from build123d import *

# Parameters (mm, degrees)
F0_W     = 105
F0_H     = 50
F0_R     = 6
F1_DEPTH = 15
F2_R     = 3
F3_DEPTH = 15
F4_R     = 2.6
F5_DEPTH = 15


with BuildPart() as f1:
    # F0 (on Front) → F1 (new body)
    with BuildSketch(Plane.XZ):
        with Locations((52.5, 25)):
            Rectangle(F0_W, F0_H)
        with Locations((14, 12.5)):
            Circle(F0_R, mode=Mode.SUBTRACT)
        with Locations((91, 12.5)):
            Circle(F0_R, mode=Mode.SUBTRACT)
        with Locations((14, 37.5)):
            Circle(F0_R, mode=Mode.SUBTRACT)
        with Locations((91, 37.5)):
            Circle(F0_R, mode=Mode.SUBTRACT)
    extrude(amount=F1_DEPTH)

    # F2 (on face) → F3 (cut, through all)
    with BuildSketch(Plane.XZ.offset(15)):
        with Locations((30, 37.5)):
            Circle(F2_R)
        with Locations((75, 37.5)):
            Circle(F2_R)
        with Locations((30, 12.5)):
            Circle(F2_R)
        with Locations((75, 12.5)):
            Circle(F2_R)
    extrude(amount=-F3_DEPTH, mode=Mode.SUBTRACT)

    # F4 (on face) → F5 (cut, through all)
    with BuildSketch(Plane.XZ.offset(15)):
        with Locations((5, 45)):
            Circle(F4_R)
        with Locations((100, 45)):
            Circle(F4_R)
        with Locations((100, 5)):
            Circle(F4_R)
        with Locations((5, 5)):
            Circle(F4_R)
    extrude(amount=-F5_DEPTH, mode=Mode.SUBTRACT)


solid = f1.part
Check sheet for the modelled part. Datum: model origin and axes. Units: mm. Give positions to 0.01 mm unless a question says otherwise; leave off trailing zeros. Write each loop counter-clockwise with the first axis right and the second up, starting at its lowest first coordinate (ties: lowest second). Pieces come first, ordered by that corner, then holes. Notation, with made-up numbers: (71, 51.5) -> (117, 51.5) arc R22 ccw to (117, 71.5) -> close; hole circle Ø4 at (84.5, 79.25). An arc over 180 degrees is marked (long way). Use one line per item in the form item = value. Start each with the question number.
1. Section check C-C (z = 45). Record the cut outline in (x, y).
2. Thickness scan on line 1 along Z through (x, y) = (5, -6.5); line 2 along Z through (x, y) = (14, -11); line 3 along X through (y, z) = (-4.5, 6). Record the ranges inside material, lowest first. Write a range as from..to.
3. Go/stop test with flat-tipped pins: P1, Ø19, axis at x = 14, z = 12.5, coming from the -Y side; P2, Ø4.5, axis at x = 5, z = 45, coming from the +Y side. Record where each tip stops, or that it passes through.
4. Mould release check, pull along Z, two halves, no side actions. Record for faces 1 (the flat face through (52, -7, 50)), 2 (the cylindrical face through (4.662, -7.605, 7.578)), 3 (the flat face through (52, 0, 25)): pulls with the +Z half, pulls with the -Z half, needs draft (parallel to the pull), parting line crosses it, or undercut.
5. Section check B-B (x = 14). Record the cut outline in (y, z), and give its area (3 significant figures).
6. Section check A-A (z = 37.5). Record the cut outline in (x, y).
7. Section check D-D (y = -2.5). Count the separate pieces of the cut face and the enclosed holes in it, and give its area (3 significant figures).
Conclusion:
q1.outline = (0, -15) -> (2.4, -15) -> (2.4, 0) -> (0, 0) -> close; (7.6, -15) -> (97.4, -15) -> (97.4, 0) -> (7.6, 0) -> close; (102.6, -15) -> (105, -15) -> (105, 0) -> (102.6, 0) -> close
q2.line_1 = 0..2.4, 7.6..42.4, 47.6..50
q2.line_2 = 0..6.5, 18.5..31.5, 43.5..50
q2.line_3 = 0..2.6, 7.4..97.6, 102.4..105
q3.P1 = -15
q3.P2 = through
q4.face_1 = pulls with the +Z half
q4.face_2 = undercut
q4.face_3 = needs draft
q5.outline = (-15, 0) -> (0, 0) -> (0, 6.5) -> (-15, 6.5) -> close; (-15, 18.5) -> (0, 18.5) -> (0, 31.5) -> (-15, 31.5) -> close; (-15, 43.5) -> (0, 43.5) -> (0, 50) -> (-15, 50) -> close
q5.area = 390 mm²
q6.outline = (0, -15) -> (8, -15) -> (8, 0) -> (0, 0) -> close; (20, -15) -> (27, -15) -> (27, 0) -> (20, 0) -> close; (33, -15) -> (72, -15) -> (72, 0) -> (33, 0) -> close; (78, -15) -> (85, -15) -> (85, 0) -> (78, 0) -> close; (97, -15) -> (105, -15) -> (105, 0) -> (97, 0) -> close
q7.separate_pieces = 1
q7.enclosed_holes = 12
q7.area = 4,600 mm²
